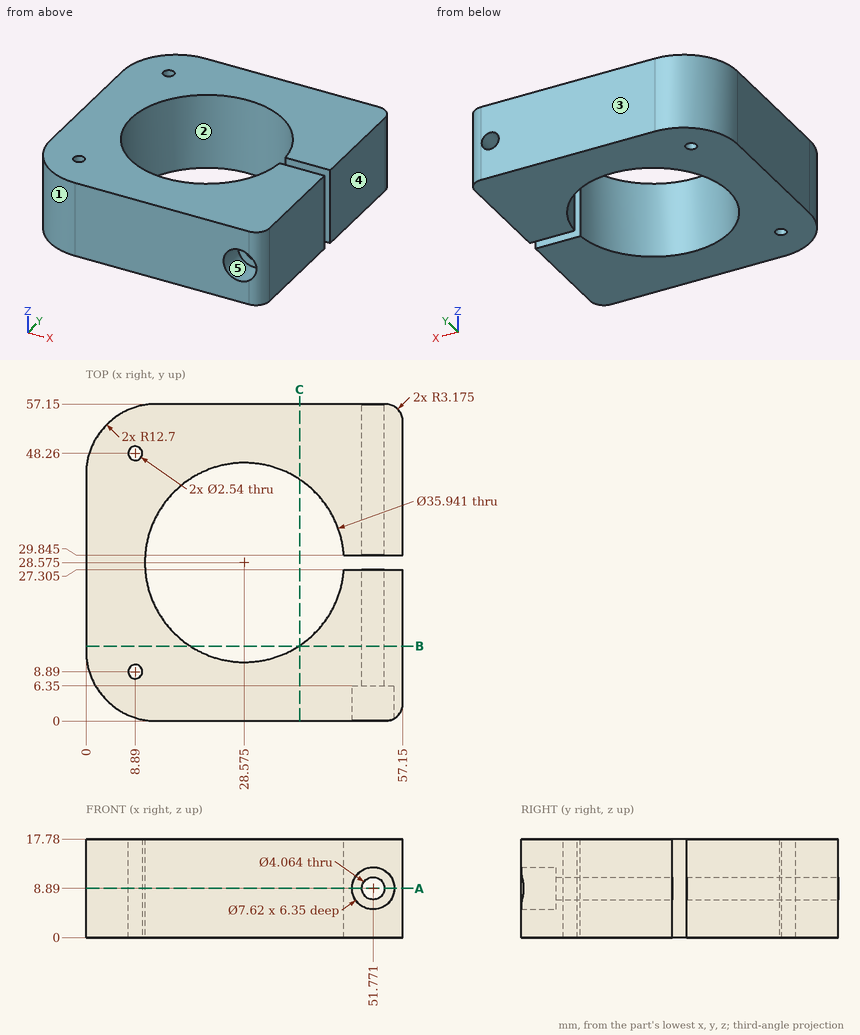
Design review of the part shown in the three views and the two pictorial views. Dimensions are in mm from the part's minimum x, y and z. A direction names the side the tool comes from. Round coordinates to 2 decimals unless told otherwise and drop trailing zeros. Write each loop counter-clockwise with the first axis right and the second up, starting at its lowest first coordinate (ties: lowest second). Pieces come first, ordered by that corner, then holes.
Item 1: For probe 1 along Y at (x, z) = (47.5, 4.5) (3 decimals); probe 2 along Y at (x, z) = (8.89, 8.25) (1 decimal); probe 3 along Y at (x, z) = (24, 16.25), list the stretches that pass through material, from the lowest coordinate up.
Item 2: Clearance check with flat-ended pins moving along their axes: pin 1 Ø2.5 at (x, z) = (50, 8) entering from -Y; pin 2 Ø6 at (x, z) = (6, 3.5) entering from -Y. State where each tip first meets the part, or that it passes through.
Item 3: The part is to be moulded in two halves that separate along X. For the marked faces 1, 2 and 3, say which applies: +X half, -X half, draft (parallel to the pull), parting line (faces both ways), or undercut.
Item 4: For the marked faces 4 and 5, list the 3-axis set-ups (+Z, -Z, +X, -X, +Y, -Y) from which the entire face can be reached by the end or side of a thin tool; tool diameter is ignored.
Item 5: We need section A-A on z = 8.89. State how many separate pieces and enclosed holes the cut face has, and give its area (3 significant figures).
Item 6: We need section B-B on y = 13.5. Write out the cut boundary in (x, z), and give its area (3 significant figures).
Item 7: We need section C-C on x = 38.5. Write out the cut boundary in (y, z).
Returned:
1. probe 1: y = 0 to 27.305, 29.845 to 57.15
1. probe 2: y = 0.6 to 7.6, 10.2 to 47, 49.5 to 56.6
1. probe 3: y = 0 to 11.2, 45.95 to 57.15
2. pin 1: stops at y = 6.35
2. pin 2: stops at y = 0.55
3. face 1: -X half
3. face 2: undercut
3. face 3: draft
4. face 4: +Z, -Z, +X, +Y, -Y
4. face 5: -Y
5. separate pieces: 3
5. enclosed holes: 2
5. area: 1,900 mm2
6. outline: (0, 0) - (18.79, 0) - (18.79, 17.78) - (0, 17.78) - close; (38.36, 0) - (57.15, 0) - (57.15, 17.78) - (38.36, 17.78) - close; hole circle Ø4.06 at (51.77, 8.89)
6. area: 655 mm2
7. outline: (0, 0) - (13.59, 0) - (13.59, 17.78) - (0, 17.78) - close; (43.56, 0) - (57.15, 0) - (57.15, 17.78) - (43.56, 17.78) - close
